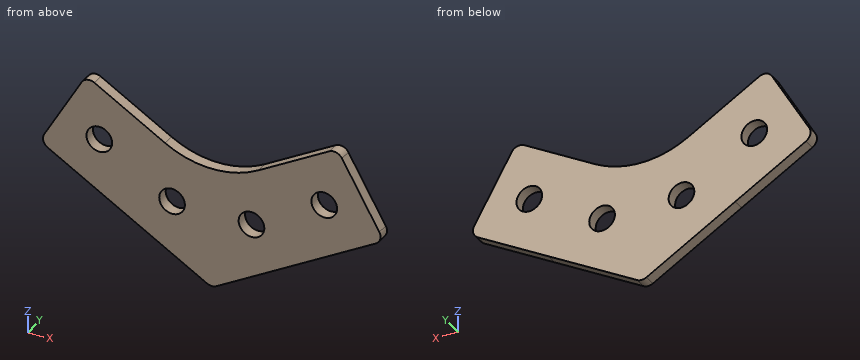
from build123d import *

# Parameters (mm, degrees)
BOSS_EXTRUDE1_DEPTH = 3.175
SKETCH2_R           = 3.4925
CUT_EXTRUDE2_DEPTH  = 3.175
LPATTERN5_COUNT     = 2
LPATTERN5_PITCH     = 22.86
SKETCH7_R           = 3.4925
CUT_EXTRUDE3_DEPTH  = 3.175
LPATTERN6_COUNT     = 2
LPATTERN6_PITCH     = 22.86
FILLET1_R           = 2.54
FILLET2_R           = 25.4


with BuildPart() as part:
    # Sketch1 → Boss-Extrude1 (new body)
    with BuildSketch(Plane(origin=(0, 0, 0), x_dir=(1, 0, 0), z_dir=(0, 1, 0))):
        Polygon((-25.4, 14.664696837), (0, 29.329393675), (25.4, 14.664696837), (46.85041276, 2.280295256), (34.15041276, -19.71675), (0, 0), (-34.15041276, -19.71675), (-46.85041276, 2.280295256), align=None)
    extrude(amount=BOSS_EXTRUDE1_DEPTH)

    # Sketch2 → Cut-Extrude2 (cut)
    with BuildSketch(Plane(origin=(0, 3.175, 0), x_dir=(1, 0, 0), z_dir=(0, 1, 0))):
        with Locations(Location((-30.601742395, -3.003227372, 0), (0, 0, 270))):
            Circle(SKETCH2_R)
    cut_extrude2 = extrude(amount=-CUT_EXTRUDE2_DEPTH, mode=Mode.SUBTRACT)

    # LPattern5: Cut-Extrude2 ×2
    with Locations(*[Vector(0.8660254037844385, 0, -0.5000000000000003) * (i * LPATTERN5_PITCH) for i in range(1, LPATTERN5_COUNT)]):
        add(cut_extrude2, mode=Mode.SUBTRACT)

    # Sketch7 → Cut-Extrude3 (cut)
    with BuildSketch(Plane(origin=(0, 3.175, 0), x_dir=(1, 0, 0), z_dir=(0, 1, 0))):
        with Locations(Location((30.601742395, -3.003227372, 0), (0, 0, 270))):
            Circle(SKETCH7_R)
    cut_extrude3 = extrude(amount=-CUT_EXTRUDE3_DEPTH, mode=Mode.SUBTRACT)

    # LPattern6: Cut-Extrude3 ×2
    with Locations(*[Vector(-0.8660254037844378, 0, -0.5000000000000017) * (i * LPATTERN6_PITCH) for i in range(1, LPATTERN6_COUNT)]):
        add(cut_extrude3, mode=Mode.SUBTRACT)

    # Fillet1
    fillet1_edges = [part.edges().sort_by_distance(p)[0] for p in [
        (0, 1.5875, -29.329393675),
        (46.85041276, 1.5875, -2.280295256),
        (34.15041276, 1.5875, 19.71675),
        (-34.15041276, 1.5875, 19.71675),
        (-46.85041276, 1.5875, -2.280295256),
    ]]
    fillet(fillet1_edges, radius=FILLET1_R)

    # Fillet2
    fillet2_edges = [part.edges().sort_by_distance(p)[0] for p in [
        (0, 1.5875, 0),
    ]]
    fillet(fillet2_edges, radius=FILLET2_R)


solid = part.part
Geometry check sheet. Reference: the model listing, model coordinates, mm. Give positions to 0.01 mm unless a question says otherwise; leave off trailing zeros. Order: outer loops, then holes, each group sorted by start corner. A loop starts at its lowest first (then second) coordinate and runs counter-clockwise, first axis right, second up.
1) Cross-section at B-B (x = -28.5). Record the boundary of the cut face in (y, z) (3 decimals).
Results are:
outline: (0, -12.875) - (3.175, -12.875) - (3.175, 0.214) - (0, 0.214) - close; (0, 5.793) - (3.175, 5.793) - (3.175, 16.454) - (0, 16.454) - close
2) Cross-section at C-C (y = 1.2). Record the boundary of the cut face in (x, z) (1 decimal).
Results are:
outline: (-45.6, -0.1) arc R2.5 ccw to (-44.7, -3.6) - (-1.3, -28.6) arc R2.5 ccw to (1.3, -28.6) - (44.7, -3.6) arc R2.5 ccw to (45.6, -0.1) - (35.4, 17.5) arc R2.5 ccw to (32, 18.4) - (12.7, 7.3) arc R25.4 cw to (-12.7, 7.3) - (-32, 18.4) arc R2.5 ccw to (-35.4, 17.5) - close; hole circle Ø7 at (-30.6, 3); hole circle Ø7 at (-10.8, -8.4); hole circle Ø7 at (10.8, -8.4); hole circle Ø7 at (30.6, 3)
3) Material ranges on probe 1 along X at (y, z) = (2, 6); probe 2 along X at (y, z) = (1.55, -10); probe 3 along X at (y, z) = (0.4, -9.5), recorded low to high.
Results are:
probe 1: x = -42.07 to -32.4, -28.81 to -10.04, 10.04 to 28.81, 32.4 to 42.07
probe 2: x = -33.48 to -13.92, -7.69 to 7.69, 13.92 to 33.48
probe 3: x = -34.35 to -14.13, -7.48 to 7.48, 14.13 to 34.35
4) Cross-section at D-D (z = 2.5). Record the boundary of the cut face in (x, y) (1 decimal), then the cut area to 3 significant figures.
Results are:
outline: (-44.1, 0) - (-34.1, 0) - (-34.1, 3.2) - (-44.1, 3.2) - close; (-27.1, 0) - (27.1, 0) - (27.1, 3.2) - (-27.1, 3.2) - close; (34.1, 0) - (44.1, 0) - (44.1, 3.2) - (34.1, 3.2) - close
area: 236 mm2
5) Gauge pin test, flat end, axial feed: pin 1 (5.5 mm diameter, centred on x = -10.8, z = -8.43, fed in from +Y). Record the tip position at first contact, or that the pin passes through.
Results are:
pin 1: passes through
6) Cross-section at A-A (z = 9.5). Record the boundary of the cut face in (x, y) (3 decimals).
Results are:
outline: (-40.049, 0) - (-16.454, 0) - (-16.454, 3.175) - (-40.049, 3.175) - close; (16.454, 0) - (40.049, 0) - (40.049, 3.175) - (16.454, 3.175) - close
